Read the model definition and answer for the solid it produces. Units are mm, in the model's axes. A direction names the side the tool comes from. Give positions to 0.01 mm unless a question says otherwise; leave off trailing zeros. Order: outer loops, then holes, each group sorted by start corner. A loop starts at its lowest first (then second) coordinate and runs counter-clockwise, first axis right, second up. Notation, with made-up numbers: M 53,-39.75 L 104,-39.75 A27 cw 104,-9.75 Z; hole C -5,41.25 d9. An arc over 180 degrees is marked long. Write item = value, one per line. Start each with the question number.
from build123d import *

# Parameters (mm, degrees)
F0_W     = 233.391122
F0_H     = 167.760142
F0_R     = 14.287094
F0_R_2   = 14.2875
F0_R_3   = 14.287856
F0_R_4   = 14.261292
F0_R_5   = 14.287475
F0_R_6   = 12.700237
F1_DEPTH = 2.5
F2_W     = 3
F2_H     = 3
F2_W_2   = 227.391122
F2_H_2   = 161.760142
F3_DEPTH = 2.5


with BuildPart() as f1:
    # F0 (on Front) → F1 (new body)
    with BuildSketch(Plane.XZ):
        Rectangle(F0_W, F0_H)
        with Locations((-17.460909, -51.958768)):
            Circle(F0_R, mode=Mode.SUBTRACT)
        with Locations((20.706644, -51.958057)):
            Circle(F0_R_2, mode=Mode.SUBTRACT)
        with Locations((2.589838, -16.863295)):
            Circle(F0_R, mode=Mode.SUBTRACT)
        with Locations((40.757772, -16.864183)):
            Circle(F0_R_3, mode=Mode.SUBTRACT)
        with Locations((78.93528, -16.822839)):
            Circle(F0_R_4, mode=Mode.SUBTRACT)
        with Locations((-68.03398, 19.30053)):
            Circle(F0_R_5, mode=Mode.SUBTRACT)
        with Locations((-17.608788, 58.596443)):
            Circle(F0_R_6, mode=Mode.SUBTRACT)
        with Locations((2.591311, 18.233144)):
            Circle(F0_R_2, mode=Mode.SUBTRACT)
        with Locations((40.755791, 18.233144)):
            Circle(F0_R_2, mode=Mode.SUBTRACT)
        with Locations((78.921871, 18.233144)):
            Circle(F0_R_2, mode=Mode.SUBTRACT)
        with Locations((20.70639, 58.596469)):
            Circle(F0_R_6, mode=Mode.SUBTRACT)
    extrude(amount=F1_DEPTH)

    # F2 (on face) → F3 (join)
    with BuildSketch(Plane(origin=(0, 0, 0), x_dir=(-1, 0, 0), z_dir=(0, 1, 0))):
        with Locations((-115.195561, -82.380071)):
            Rectangle(F2_W, F2_H)
        with Locations((0, -82.380071)):
            Rectangle(F2_W_2, F2_H)
        with Locations((-115.195561, 0)):
            Rectangle(F2_W, F2_H_2)
        with Locations((115.195561, -82.380071)):
            Rectangle(F2_W, F2_H)
        with Locations((-115.195561, 82.380071)):
            Rectangle(F2_W, F2_H)
        with Locations((115.195561, 0)):
            Rectangle(F2_W, F2_H_2)
        with Locations((0, 82.380071)):
            Rectangle(F2_W_2, F2_H)
        with Locations((115.195561, 82.380071)):
            Rectangle(F2_W, F2_H)
    extrude(amount=F3_DEPTH)


solid = f1.part
1) For faces 5 (the face through (-2, 0, 1)), 6 (the face through (0.5, 2.5, 81.2)), determine the directions among +Z, -Z, +X, -X, +Y, -Y from which every point of the face is accessible in a straight line to the end or side of a thin tool.
2) Find the intervals of material crossed by probe 1 along X at (y, z) = (2, 60.5); probe 2 along Z at (x, y) = (36, 2.05); probe 3 along X at (y, z) = (-1.5, 6.5), in increasing order. Write a range as [from, to].
3) Find section A-A on x = 76. Determine the outline of the cut face in (y, z), plus the area to 3 significant figures.
4) Find section B-B on z = -48. Determine the outline of the cut face in (x, y), plus the area to 3 significant figures.
5) This flat-tipped pin is pushed along its axis until it touches: P1, Ø4, axis at x = -85.5, z = -61, coming from the +Y side. Where does it stop, or does it pass through?
6) For a pull along Z with two mould halves and no side action, classify faces 1 (the face through (-2, 0, 83.88)), 2 (the face through (-19.26, -1.23, 71.19)), 3 (the face through (-116.696, 0, -1)), 4 (the face through (2, 0, -83.88)) as pulls with the +Z half, pulls with the -Z half, needs draft (parallel to the pull), parting line crosses it, or undercut.
7) Find section D-D on z = 28.5. Determine the outline of the cut face in (x, y), plus the area to 3 significant figures.
8) Find section C-C on y = -1.4. Count the separate pieces of the cut face and the enclosed holes in it, plus the area to 3 significant figures.
Numbers:
q1.face_5 = +Y
q1.face_6 = +Z, -Z, +X, -X, +Y
q2.probe_1 = [-116.7, -113.7], [113.7, 116.7]
q2.probe_2 = [-83.88, -80.88], [80.88, 83.88]
q2.probe_3 = [-116.7, -74.38], [-61.69, -5.56], [10.74, 32.6], [48.91, 70.77], [87.07, 116.7]
q3.outline = M -2.5,-83.88 L 2.5,-83.88 L 2.5,-80.88 L 0,-80.88 L 0,-30.78 L -2.5,-30.78 Z; M -2.5,-2.87 L 0,-2.87 L 0,4.25 L -2.5,4.25 Z; M -2.5,32.22 L 0,32.22 L 0,80.88 L 2.5,80.88 L 2.5,83.88 L -2.5,83.88 Z
q3.area = 295 mm2
q4.outline = M -116.7,-2.5 L -31.19,-2.5 L -31.19,0 L -113.7,0 L -113.7,2.5 L -116.7,2.5 Z; M -3.73,-2.5 L 6.98,-2.5 L 6.98,0 L -3.73,0 Z; M 34.43,-2.5 L 116.7,-2.5 L 116.7,2.5 L 113.7,2.5 L 113.7,0 L 34.43,0 Z
q4.area = 461 mm2
q5.P1 = 0
q6.face_1 = pulls with the +Z half
q6.face_2 = undercut
q6.face_3 = needs draft
q6.face_4 = pulls with the -Z half
q7.outline = M -116.7,-2.5 L -78.97,-2.5 L -78.97,0 L -113.7,0 L -113.7,2.5 L -116.7,2.5 Z; M -57.1,-2.5 L -7.34,-2.5 L -7.34,0 L -57.1,0 Z; M 12.53,-2.5 L 30.82,-2.5 L 30.82,0 L 12.53,0 Z; M 50.69,-2.5 L 68.99,-2.5 L 68.99,0 L 50.69,0 Z; M 88.86,-2.5 L 116.7,-2.5 L 116.7,2.5 L 113.7,2.5 L 113.7,0 L 88.86,0 Z
q7.area = 395 mm2
q8.separate_pieces = 1
q8.enclosed_holes = 11
q8.area = 32,400 mm2
